Could you check a few things on this model? Use its own coordinates, in mm. Give positions to 0.01 mm unless a question says otherwise; leave off trailing zeros. Order: outer loops, then holes, each group sorted by start corner. A loop starts at its lowest first (then second) coordinate and runs counter-clockwise, first axis right, second up.
from build123d import *

# Parameters (mm, degrees)
F2_DEPTH = 25.4
F3_SIZE  = 5.08


with BuildPart() as f2:
    # F1 (on face) → F2 (new body)
    with BuildSketch(Plane.XY):
        Polygon((15.33778, 23.638219), (55.396467, 38.976014), (34.645349, 65.320902), align=None)
    extrude(amount=F2_DEPTH)

    # F3
    f3_edges = [f2.edges().sort_by_distance(p)[0] for p in [
        (45.020908, 52.148458, 25.4),
        (24.991564, 44.47956, 25.4),
        (35.367124, 31.307116, 25.4),
    ]]
    chamfer(f3_edges, length=F3_SIZE)


solid = f2.part
Item 1: Imagine slicing it at A-A on z = 13.5. List the corners of the cut face in (x, y) for me, then the cut area to 3 significant figures.
Findings:
outline: (15.34, 23.64) - (55.4, 38.98) - (34.65, 65.32) - close
area: 687 mm2
Item 2: Please list where these lines run through material, in increasing order: line 1 along Z through (x, y) = (37, 56); line 2 along Y through (x, z) = (31, 2.5); line 3 along Y through (x, z) = (48.5, 21.5).
Findings:
line 1: z = 0 to 24.24
line 2: y = 29.64 to 57.45
line 3: y = 37.6 to 45.82
Item 3: For pin 1 (5 mm diameter, centred on x = 27.5, z = 18, fed in from +Y); pin 2 (1.5 mm diameter, centred on y = 59.5, z = 12.5, fed in from +X); pin 3 (1.5 mm diameter, centred on y = 42.5, z = 19, fed in from -X), each with a flat end and sliding along its axis, tell me the tip position at first contact or that it passes through.
Findings:
pin 1: stops at y = 55.29
pin 2: stops at x = 39.82
pin 3: stops at x = 23.73
Item 4: Imagine slicing it at C-C on x = 41. List the corners of the cut face in (y, z) for me.
Findings:
outline: (33.46, 0) - (57.25, 0) - (57.25, 20.32) - (49.04, 25.4) - (38.9, 25.4) - (33.46, 20.32) - close
Item 5: Imagine slicing it at B-B on y = 27. List the corners of the cut face in (x, z) for me, then the cut area to 3 significant figures.
Findings:
outline: (16.89, 0) - (24.12, 0) - (24.12, 20.32) - (18.94, 22.17) - (16.89, 20.32) - close
area: 153 mm2
Item 6: Imagine slicing it at D-D on x = 52. List the corners of the cut face in (y, z) for me.
Findings:
outline: (37.68, 0) - (43.29, 0) - (43.29, 20.32) - (39.91, 22.41) - (37.68, 20.32) - close
